```python
from build123d import *

# Parameters (mm, degrees)
SKETCH2_R                    = 1.425
BOSS_EXTRUDE1_DEPTH          = 3.175
SKETCH3_R                    = 2.5
CUT_EXTRUDE1_DEPTH           = 0.5
SKETCH4_R                    = 2.5
CUT_EXTRUDE2_DEPTH           = 1.2
CUT_EXTRUDE2_DRAFT           = -42
CUT_EXTRUDE2_PROFILE_2_DEPTH = 1.2
CUT_EXTRUDE2_PROFILE_2_DRAFT = -42
CUT_EXTRUDE2_PROFILE_3_DEPTH = 1.2
CUT_EXTRUDE2_PROFILE_3_DRAFT = -42
CUT_EXTRUDE2_PROFILE_4_DEPTH = 1.2
CUT_EXTRUDE2_PROFILE_4_DRAFT = -42
CUT_EXTRUDE2_PROFILE_5_DEPTH = 1.2
CUT_EXTRUDE2_PROFILE_5_DRAFT = -42
CUT_EXTRUDE2_PROFILE_6_DEPTH = 1.2
CUT_EXTRUDE2_PROFILE_6_DRAFT = -42


with BuildPart() as part:
    # Sketch2 → Boss-Extrude1 (new body)
    with BuildSketch(Plane(origin=(0, 0, 0), x_dir=(1, 0, 0), z_dir=(0, 1, 0))):
        with BuildLine():
            Line((-145.18277075, -44.880968233), (-179.497120097, -25.768390824))
            ThreePointArc((-179.497120097, -25.768390824), (-183.588653035, -24.128556812), (-187.960968922, -23.569494069))
            Line((-187.960968922, -23.569494069), (-247.377604545, -27.068041697))
            ThreePointArc((-247.377604545, -27.068041697), (-255.760524502, -29.218913898), (-262.07032604, -35.142257782))
            ThreePointArc((-262.07032604, -35.142257782), (-266.807761783, -43.251676507), (-270.933745897, -51.688632391))
            Line((-270.933745897, -51.688632391), (-273.728235609, -57.981701498))
            ThreePointArc((-273.728235609, -57.981701498), (-274.847170355, -61.434035543), (-275.2256366, -65.043382939))
            Line((-275.2256366, -65.043382939), (-275.2256366, -88.130010281))
            ThreePointArc((-275.2256366, -88.130010281), (-270.129294593, -100.433668273), (-257.8256366, -105.530010281))
            Line((-257.8256366, -105.530010281), (-193.494425739, -105.530010281))
            ThreePointArc((-193.494425739, -105.530010281), (-186.835734016, -104.205514146), (-181.190767747, -100.433668273))
            Line((-181.190767747, -100.433668273), (-180.680815133, -99.923715659))
            ThreePointArc((-180.680815133, -99.923715659), (-176.755292612, -97.300765368), (-172.12482308, -96.379707712))
            Line((-172.12482308, -96.379707712), (-153.649556898, -96.379707712))
            ThreePointArc((-153.649556898, -96.379707712), (-141.345898905, -91.283365704), (-136.249556898, -78.979707712))
            Line((-136.249556898, -78.979707712), (-136.249556898, -73.280889471))
            Line((-136.249556898, -73.280889471), (-138.999556898, -73.280889471))
            Line((-138.999556898, -73.280889471), (-138.999556898, -65.780889471))
            Line((-138.999556898, -65.780889471), (-136.249556898, -65.780889471))
            Line((-136.249556898, -65.780889471), (-136.249556898, -60.08207123))
            ThreePointArc((-136.249556898, -60.08207123), (-138.648188978, -51.266235449), (-145.18277075, -44.880968233))
        make_face()
        with Locations(Location((-147.207602145, -91.127288498, 0), (0, 0, 270))):
            Circle(SKETCH2_R, mode=Mode.SUBTRACT)
        with Locations(Location((-141.795027651, -53.115534334, 0), (0, 0, 270))):
            Circle(SKETCH2_R, mode=Mode.SUBTRACT)
        with Locations(Location((-187.963906245, -27.219493821, 0), (0, 0, 270))):
            Circle(SKETCH2_R, mode=Mode.SUBTRACT)
        with Locations(Location((-253.051529835, -31.941972813, 0), (0, 0, 270))):
            Circle(SKETCH2_R, mode=Mode.SUBTRACT)
        with Locations(Location((-267.548354841, -97.852728522, 0), (0, 0, 270))):
            Circle(SKETCH2_R, mode=Mode.SUBTRACT)
        with Locations(Location((-202.85468144, -101.880010281, 0), (0, 0, 270))):
            Circle(SKETCH2_R, mode=Mode.SUBTRACT)
    extrude(amount=BOSS_EXTRUDE1_DEPTH)

    # Sketch3 → Cut-Extrude1 (cut)
    with BuildSketch(Plane(origin=(0, 3.175, 0), x_dir=(1, 0, 0), z_dir=(0, 1, 0))):
        with Locations(Location((-253.051529835, -31.941972813, 0), (0, 0, 270))):
            Circle(SKETCH3_R)
        with Locations(Location((-187.963906245, -27.219493821, 0), (0, 0, 270))):
            Circle(SKETCH3_R)
        with Locations(Location((-141.795027651, -53.115534334, 0), (0, 0, 270))):
            Circle(SKETCH3_R)
        with Locations(Location((-147.207602145, -91.127288498, 0), (0, 0, 270))):
            Circle(SKETCH3_R)
        with Locations(Location((-202.85468144, -101.880010281, 0), (0, 0, 270))):
            Circle(SKETCH3_R)
        with Locations(Location((-267.548354841, -97.852728522, 0), (0, 0, 270))):
            Circle(SKETCH3_R)
    extrude(amount=-CUT_EXTRUDE1_DEPTH, mode=Mode.SUBTRACT)


with BuildPart() as cut_extrude2_tool:
    # Sketch4 → Cut-Extrude2 (with draft: the straight prism first)
    with BuildSketch(Plane(origin=(0, 2.675, 0), x_dir=(1, 0, 0), z_dir=(0, 1, 0))):
        with Locations(Location((-267.548354841, -97.852728522, 0), (0, 0, 270))):
            Circle(SKETCH4_R)
    extrude(amount=-CUT_EXTRUDE2_DEPTH)
    # Cut-Extrude2: the draft: its side faces are tilted about the plane it starts from
    cut_extrude2_sides = [cut_extrude2_tool.faces().sort_by_distance(p)[0] for p in [
        (-267.548354841, 2.075, 95.352728522),
    ]]
    draft(cut_extrude2_sides, Plane(origin=(0, 2.675, 0), x_dir=(1, 0, 0), z_dir=(0, 1, 0)), CUT_EXTRUDE2_DRAFT)


with BuildPart() as part_1:
    add(part.part)

    # Cut-Extrude2: cut by cut_extrude2_tool
    add(cut_extrude2_tool.part, mode=Mode.SUBTRACT)


with BuildPart() as cut_extrude2_profile_2_tool:
    # Sketch4 → Cut-Extrude2 profile 2 (with draft: the straight prism first)
    with BuildSketch(Plane(origin=(0, 2.675, 0), x_dir=(1, 0, 0), z_dir=(0, 1, 0))):
        with Locations(Location((-202.85468144, -101.880010281, 0), (0, 0, 270))):
            Circle(SKETCH4_R)
    extrude(amount=-CUT_EXTRUDE2_PROFILE_2_DEPTH)
    # Cut-Extrude2 profile 2: the draft: its side faces are tilted about the plane it starts from
    cut_extrude2_profile_2_sides = [cut_extrude2_profile_2_tool.faces().sort_by_distance(p)[0] for p in [
        (-202.85468144, 2.075, 99.380010281),
    ]]
    draft(cut_extrude2_profile_2_sides, Plane(origin=(0, 2.675, 0), x_dir=(1, 0, 0), z_dir=(0, 1, 0)), CUT_EXTRUDE2_PROFILE_2_DRAFT)


with BuildPart() as part_2:
    add(part_1.part)

    # Cut-Extrude2 profile 2: cut by cut_extrude2_profile_2_tool
    add(cut_extrude2_profile_2_tool.part, mode=Mode.SUBTRACT)


with BuildPart() as cut_extrude2_profile_3_tool:
    # Sketch4 → Cut-Extrude2 profile 3 (with draft: the straight prism first)
    with BuildSketch(Plane(origin=(0, 2.675, 0), x_dir=(1, 0, 0), z_dir=(0, 1, 0))):
        with Locations(Location((-147.207602145, -91.127288498, 0), (0, 0, 270))):
            Circle(SKETCH4_R)
    extrude(amount=-CUT_EXTRUDE2_PROFILE_3_DEPTH)
    # Cut-Extrude2 profile 3: the draft: its side faces are tilted about the plane it starts from
    cut_extrude2_profile_3_sides = [cut_extrude2_profile_3_tool.faces().sort_by_distance(p)[0] for p in [
        (-147.207602145, 2.075, 88.627288498),
    ]]
    draft(cut_extrude2_profile_3_sides, Plane(origin=(0, 2.675, 0), x_dir=(1, 0, 0), z_dir=(0, 1, 0)), CUT_EXTRUDE2_PROFILE_3_DRAFT)


with BuildPart() as part_3:
    add(part_2.part)

    # Cut-Extrude2 profile 3: cut by cut_extrude2_profile_3_tool
    add(cut_extrude2_profile_3_tool.part, mode=Mode.SUBTRACT)


with BuildPart() as cut_extrude2_profile_4_tool:
    # Sketch4 → Cut-Extrude2 profile 4 (with draft: the straight prism first)
    with BuildSketch(Plane(origin=(0, 2.675, 0), x_dir=(1, 0, 0), z_dir=(0, 1, 0))):
        with Locations(Location((-141.795027651, -53.115534334, 0), (0, 0, 270))):
            Circle(SKETCH4_R)
    extrude(amount=-CUT_EXTRUDE2_PROFILE_4_DEPTH)
    # Cut-Extrude2 profile 4: the draft: its side faces are tilted about the plane it starts from
    cut_extrude2_profile_4_sides = [cut_extrude2_profile_4_tool.faces().sort_by_distance(p)[0] for p in [
        (-141.795027651, 2.075, 50.615534334),
    ]]
    draft(cut_extrude2_profile_4_sides, Plane(origin=(0, 2.675, 0), x_dir=(1, 0, 0), z_dir=(0, 1, 0)), CUT_EXTRUDE2_PROFILE_4_DRAFT)


with BuildPart() as part_4:
    add(part_3.part)

    # Cut-Extrude2 profile 4: cut by cut_extrude2_profile_4_tool
    add(cut_extrude2_profile_4_tool.part, mode=Mode.SUBTRACT)


with BuildPart() as cut_extrude2_profile_5_tool:
    # Sketch4 → Cut-Extrude2 profile 5 (with draft: the straight prism first)
    with BuildSketch(Plane(origin=(0, 2.675, 0), x_dir=(1, 0, 0), z_dir=(0, 1, 0))):
        with Locations(Location((-187.963906245, -27.219493821, 0), (0, 0, 270))):
            Circle(SKETCH4_R)
    extrude(amount=-CUT_EXTRUDE2_PROFILE_5_DEPTH)
    # Cut-Extrude2 profile 5: the draft: its side faces are tilted about the plane it starts from
    cut_extrude2_profile_5_sides = [cut_extrude2_profile_5_tool.faces().sort_by_distance(p)[0] for p in [
        (-187.963906245, 2.075, 24.719493821),
    ]]
    draft(cut_extrude2_profile_5_sides, Plane(origin=(0, 2.675, 0), x_dir=(1, 0, 0), z_dir=(0, 1, 0)), CUT_EXTRUDE2_PROFILE_5_DRAFT)


with BuildPart() as part_5:
    add(part_4.part)

    # Cut-Extrude2 profile 5: cut by cut_extrude2_profile_5_tool
    add(cut_extrude2_profile_5_tool.part, mode=Mode.SUBTRACT)


with BuildPart() as cut_extrude2_profile_6_tool:
    # Sketch4 → Cut-Extrude2 profile 6 (with draft: the straight prism first)
    with BuildSketch(Plane(origin=(0, 2.675, 0), x_dir=(1, 0, 0), z_dir=(0, 1, 0))):
        with Locations(Location((-253.051529835, -31.941972813, 0), (0, 0, 270))):
            Circle(SKETCH4_R)
    extrude(amount=-CUT_EXTRUDE2_PROFILE_6_DEPTH)
    # Cut-Extrude2 profile 6: the draft: its side faces are tilted about the plane it starts from
    cut_extrude2_profile_6_sides = [cut_extrude2_profile_6_tool.faces().sort_by_distance(p)[0] for p in [
        (-253.051529835, 2.075, 29.441972813),
    ]]
    draft(cut_extrude2_profile_6_sides, Plane(origin=(0, 2.675, 0), x_dir=(1, 0, 0), z_dir=(0, 1, 0)), CUT_EXTRUDE2_PROFILE_6_DRAFT)


with BuildPart() as part_6:
    add(part_5.part)

    # Cut-Extrude2 profile 6: cut by cut_extrude2_profile_6_tool
    add(cut_extrude2_profile_6_tool.part, mode=Mode.SUBTRACT)


solid = part_6.part
```
Work out the finished part from the listing and answer in its coordinate system (mm). A direction names the side the tool comes from. Coordinates: 2 decimals unless noted, no trailing zeros. Write each loop counter-clockwise with the first axis right and the second up, starting at its lowest first coordinate (ties: lowest second). Pieces come first, ordered by that corner, then holes. Notation, with made-up numbers: (73.5, 78) - (120.5, 78) arc R25 ccw to (120.5, 101) - close; hole circle Ø6 at (66.25, -38). An arc over 180 degrees is marked (long way). Answer as a JSON object with one key per item and string values.
Q1. Find section A-A (z = 68). Write down the section's boundary in (x, y) (3 decimals), plus the area to 3 significant figures.
Results list:
{"outline": "(-275.226, 0) - (-139, 0) - (-139, 3.175) - (-275.226, 3.175) - close", "area": "433 mm^2"}
Q2. Given pin 1 Ø4.5 at (x, z) = (-202.85, 101.88) entering from +Y; pin 2 Ø0.8 at (x, y) = (-137.5, 1) entering from +Z; pin 3 Ø1.4 at (x, y) = (-137, 1) entering from -Z, each flat-ended and moving along its own axis, determine where each tip first touches the part or whether it passes through.
Results list:
{"pin 1": "stops at y = 2.4", "pin 2": "stops at z = 86.38", "pin 3": "stops at z = 53.13"}
Q3. Find section C-C (x = -156.5). Write down the section's boundary in (y, z) (3 decimals).
Results list:
{"outline": "(0, 38.577) - (3.175, 38.577) - (3.175, 96.38) - (0, 96.38) - close"}
Q4. Which of the six approach directions +Z, -Z, +X, -X, +Y, -Y give full straight-line access (tool end or side, diameter ignored) to faces 5 (the flat face through (-163, 2, 96.38)), 6 (the flat face through (-139, 2, 70)), 7 (the cylindrical face through (-183.529, 1.565, 24.144)), 8 (the cylindrical face through (-205.073, 2.928, 103.034))?
Results list:
{"face 5": "+Z, +X, +Y, -Y", "face 6": "+X, +Y, -Y", "face 7": "-Z, +X, +Y, -Y", "face 8": "+Y"}
Q5. Consider L1, parallel to X at y = 2.6, z = 64; L2, parallel to X at y = 1.85, z = 53; L3, parallel to Z at x = -252, y = 1.25. Determine where each line is inside the solid, lowest interval first. Write a range as from..to.
Results list:
{"L1": "x = -275.19..-136.25", "L2": "x = -271.52..-143.55, -140.04..-137.76", "L3": "z = 27.69..30.98, 32.9..105.53"}
Q6. Find section B-B (y = 0.95). State how many separate pieces and enclosed holes the cut face has, plus the area to 3 significant figures.
Results list:
{"separate pieces": "1", "enclosed holes": "6", "area": "9,640 mm^2"}
Q7. For a pull along X with two mould halves and no side action, classify faces 1 (the flat face through (-272.31, 1.57, 54.79)), 2 (the cylindrical face through (-138.58, 1.57, 51.38)), 3 (the cylindrical face through (-269.99, 2.93, 97.31)), 4 (the flat face through (-207, 0, 64)) as pulls with the +X half, pulls with the -X half, needs draft (parallel to the pull), parting line crosses it, or undercut.
Results list:
{"face 1": "pulls with the -X half", "face 2": "pulls with the +X half", "face 3": "undercut", "face 4": "needs draft"}
